Part model, mm, in its own coordinate system. A direction names the side the tool comes from. Round coordinates to 2 decimals unless told otherwise and drop trailing zeros. Order: outer loops, then holes, each group sorted by start corner. A loop starts at its lowest first (then second) coordinate and runs counter-clockwise, first axis right, second up. Notation, with made-up numbers: (68.25, 60) - (121.25, 60) arc R30 cw to (121.25, 86) - close; hole circle Ø5 at (-5.75, -4.75). An arc over 180 degrees is marked (long way). Answer as a JSON object with one key per item and string values.
```python
from build123d import *

# Parameters (mm, degrees)
CROQUIS1_R              = 3.5
CROQUIS1_R_2            = 2
CROQUIS1_W              = 3
CROQUIS1_H              = 10
SALIENTE_EXTRUIR2_DEPTH = 3.5


with BuildPart() as part:
    # Croquis1 → Saliente-Extruir2 (new body)
    with BuildSketch(Plane.XY):
        with BuildLine():
            Line((36.805064583, 12.5), (36.805064583, -12.5))
            Line((36.805064583, -12.5), (-83.194935417, -12.5))
            ThreePointArc((-83.194935417, -12.5), (-106.486497393, 0), (-83.194935417, 12.5))
            Line((-83.194935417, 12.5), (36.805064583, 12.5))
        make_face()
        with Locations((-91.486497393, 0)):
            Circle(CROQUIS1_R, mode=Mode.SUBTRACT)
        with Locations((-72.486497393, 0)):
            Circle(CROQUIS1_R_2, mode=Mode.SUBTRACT)
        with Locations((24.805064583, 6)):
            Circle(CROQUIS1_R_2, mode=Mode.SUBTRACT)
        with Locations((24.805064583, -6)):
            Circle(CROQUIS1_R_2, mode=Mode.SUBTRACT)
        with Locations((-37.486497393, 0)):
            Circle(CROQUIS1_R_2, mode=Mode.SUBTRACT)
        with Locations((-2.486497393, 0)):
            Circle(CROQUIS1_R_2, mode=Mode.SUBTRACT)
        with Locations((12.805064583, 0)):
            Rectangle(CROQUIS1_W, CROQUIS1_H, mode=Mode.SUBTRACT)
    extrude(amount=SALIENTE_EXTRUIR2_DEPTH)


solid = part.part
```
Item 1: Cut at A-A (y = 0). Write the cut outline in (x, z), plus the area to 3 significant figures.
Taken from the geometry:
{"outline": "(-106.49, 0) - (-94.99, 0) - (-94.99, 3.5) - (-106.49, 3.5) - close; (-87.99, 0) - (-74.49, 0) - (-74.49, 3.5) - (-87.99, 3.5) - close; (-70.49, 0) - (-39.49, 0) - (-39.49, 3.5) - (-70.49, 3.5) - close; (-35.49, 0) - (-4.49, 0) - (-4.49, 3.5) - (-35.49, 3.5) - close; (-0.49, 0) - (11.31, 0) - (11.31, 3.5) - (-0.49, 3.5) - close; (14.31, 0) - (36.81, 0) - (36.81, 3.5) - (14.31, 3.5) - close", "area": "425 mm2"}
Item 2: Probe L1, parallel to X at y = 0.5, z = 0.4; L2, parallel to Y at x = -91.5, z = 0.45; L3, parallel to X at y = 3, z = 0.85. List the from-to ranges inside material, lowest first. Write a range as from..to.
Taken from the geometry:
{"L1": "-106.48..-94.95, -88.02..-74.42, -70.55..-39.42, -35.55..-4.42, -0.55..11.31, 14.31..36.81", "L2": "-15..-3.5, 3.5..15", "L3": "-106.18..-93.29, -89.68..11.31, 14.31..36.81"}
Item 3: Drop flat-ended pins along their axis: P1, Ø1.8, axis at x = -4.5, z = 2, coming from the +Y side; P2, Ø1, axis at x = -51.5, z = 2, coming from the -Y side. Give the stop position or say it passes through.
Taken from the geometry:
{"P1": "y = 12.5", "P2": "y = -12.5"}
Item 4: Tool access for faces 1 (the flat face through (13, 5, 2)), 2 (the flat face through (-24, 12.5, 2)), 3 (the flat face through (-22, -12.5, 2)), 4 (the flat face through (-34, 0, 0)), 5 (the flat face through (-34, 0, 3.5)): list every direction of +Z, -Z, +X, -X, +Y, -Y with a clear straight run to the whole face (end or side of a thin tool).
Taken from the geometry:
{"face 1": "+Z, -Z", "face 2": "+Z, -Z, +X, +Y", "face 3": "+Z, -Z, +X, -Y", "face 4": "-Z, +X, -X, +Y, -Y", "face 5": "+Z, +X, -X, +Y, -Y"}
Item 5: Cut at C-C (x = -29.5). Write the cut outline in (y, z).
Taken from the geometry:
{"outline": "(-12.5, 0) - (12.5, 0) - (12.5, 3.5) - (-12.5, 3.5) - close"}
Item 6: Cut at D-D (y = -11). Write the cut outline in (x, z).
Taken from the geometry:
{"outline": "(-101.68, 0) - (36.81, 0) - (36.81, 3.5) - (-101.68, 3.5) - close"}
Item 7: Cut at B-B (z = 2.75). Write the cut outline in (x, y), plus the area to 3 significant figures.
Taken from the geometry:
{"outline": "(-83.19, -12.5) - (36.81, -12.5) - (36.81, 12.5) - (-83.19, 12.5) arc R15 ccw (long way) to start; hole circle Ø7 at (-91.49, 0); hole circle Ø4 at (-72.49, 0); hole circle Ø4 at (-37.49, 0); hole circle Ø4 at (-2.49, 0); hole (11.31, -5) - (14.31, -5) - (14.31, 5) - (11.31, 5) - close; hole circle Ø4 at (24.81, -6); hole circle Ø4 at (24.81, 6)", "area": "3,460 mm2"}
